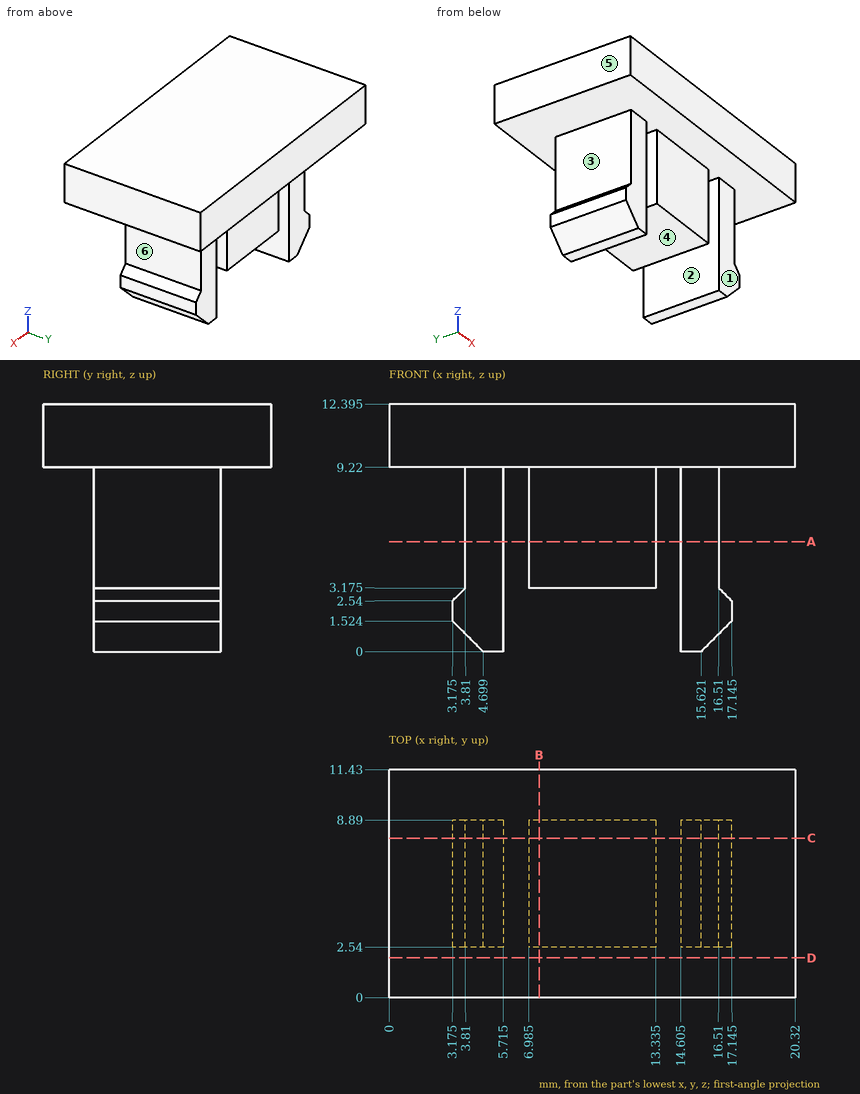
Verification items for this drawing (mm, ordinates from the low corner). A direction names the side the tool comes from. Coordinates: 2 decimals unless noted, no trailing zeros. Order: outer loops, then holes, each group sorted by start corner. A loop starts at its lowest first (then second) coordinate and runs counter-clockwise, first axis right, second up. Notation, with made-up numbers: (51.25, -17) - (71.25, -17) arc R14 cw to (71.25, 4) - close; hole circle Ø1 at (-15, 71.25). An arc over 180 degrees is marked (long way). Use one line per item in the form item = value.
1. Gauge pin test, flat ends, axial feed: pin 1 (5 mm diameter, centred on y = 5.5, z = 3.5, fed in from -X) (3 decimals); pin 2 (6 mm diameter, centred on x = 17, z = 5.5, fed in from +Y); pin 3 (5 mm diameter, centred on y = 4.5, z = 3, fed in from +X) (3 decimals). Record the tip position at first contact, or that the pin passes through.
Here are the results:
pin_1 = 3.175
pin_2 = 8.89
pin_3 = 17.145
2. Section check C-C (y = 8). Record the boundary of the cut face in (x, z) (1 decimal), then the cut area to 3 significant figures.
Here are the results:
outline = (0, 9.2) - (3.8, 9.2) - (3.8, 3.2) - (3.2, 2.5) - (3.2, 1.5) - (4.7, 0) - (5.7, 0) - (5.7, 9.2) - (7, 9.2) - (7, 3.2) - (13.3, 3.2) - (13.3, 9.2) - (14.6, 9.2) - (14.6, 0) - (15.6, 0) - (17.1, 1.5) - (17.1, 2.5) - (16.5, 3.2) - (16.5, 9.2) - (20.3, 9.2) - (20.3, 12.4) - (0, 12.4) - close
area = 139 mm²
3. Section check D-D (y = 2). Record the boundary of the cut face in (x, z) (1 decimal).
Here are the results:
outline = (0, 9.2) - (20.3, 9.2) - (20.3, 12.4) - (0, 12.4) - close
4. Section check A-A (z = 5.5). Record the boundary of the cut face in (x, y) (3 decimals), then the cut area to 3 significant figures.
Here are the results:
outline = (3.81, 2.54) - (5.715, 2.54) - (5.715, 8.89) - (3.81, 8.89) - close; (6.985, 2.54) - (13.335, 2.54) - (13.335, 8.89) - (6.985, 8.89) - close; (14.605, 2.54) - (16.51, 2.54) - (16.51, 8.89) - (14.605, 8.89) - close
area = 64.5 mm²
5. Draft check along X on the marked faces 4, 5 and 6. Enter one of: pulls with the +X half, pulls with the -X half, needs draft (parallel to the pull), parting line crosses it, or undercut.
Here are the results:
face_4 = undercut
face_5 = pulls with the -X half
face_6 = pulls with the +X half
6. Scan lines: line 1 (X direction, y = 6.5, z = 5) (3 decimals); line 2 (Z direction, x = 4.25, y = 0.5) (1 decimal); line 3 (Y direction, x = 15.25, z = 8). Record each from-to range of solid material in increasing order.
Here are the results:
line_1 = 3.81 to 5.715, 6.985 to 13.335, 14.605 to 16.51
line_2 = 9.2 to 12.4
line_3 = 2.54 to 8.89
7. Section check B-B (x = 7.5). Record the boundary of the cut face in (y, z) (1 decimal).
Here are the results:
outline = (0, 9.2) - (2.5, 9.2) - (2.5, 3.2) - (8.9, 3.2) - (8.9, 9.2) - (11.4, 9.2) - (11.4, 12.4) - (0, 12.4) - close
8. Access from +Z, -Z, +X, -X, +Y, -Y to the whole of each face (thin tool, end or side, straight path). Record for the marked faces 1, 2 and 3.
Here are the results:
face_1 = -Z, +X, -X, -Y
face_2 = -Z, +Y, -Y
face_3 = -X, +Y, -Y
